Check sheet for the modelled part. Datum: model origin and axes. Units: mm. Coordinates: 2 decimals unless noted, no trailing zeros. Loops run counter-clockwise (first coordinate to the right, second up) from the corner with the lowest first, then second, coordinate; pieces in that order, holes last.
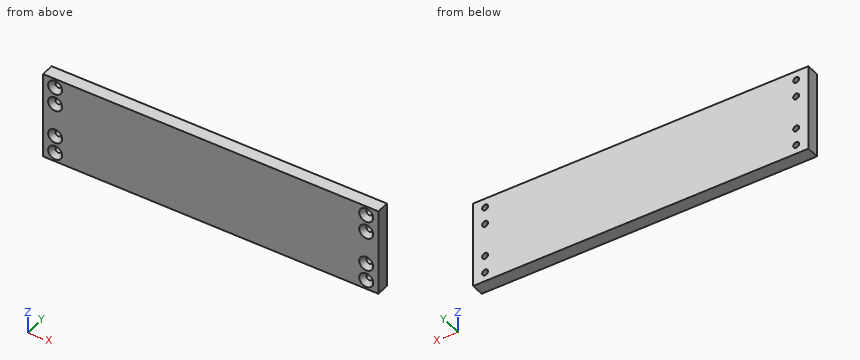
```python
from build123d import *

# Parameters (mm, degrees)
SKETCH1_W                                         = 166
SKETCH1_H                                         = 42.51
BOSS_EXTRUDE1_DEPTH                               = 6.35
F_4_CLEARANCE_HOLE1_D                             = 2.9464
CSK_FOR_4_FLAT_HEAD_SOCKET_CAP_SCREW1_D           = 2.9464
CSK_FOR_4_FLAT_HEAD_SOCKET_CAP_SCREW1_CSINK_D     = 6.9116702
CSK_FOR_4_FLAT_HEAD_SOCKET_CAP_SCREW1_CSINK_ANGLE = 82


with BuildPart() as part:
    # Sketch1 → Boss-Extrude1 (new body)
    with BuildSketch(Plane(origin=(0, 0, 0), x_dir=(1, 0, 0), z_dir=(0, 1, 0))):
        Rectangle(SKETCH1_W, SKETCH1_H)
    extrude(amount=BOSS_EXTRUDE1_DEPTH)

    # #4 Clearance Hole1 (through all)
    with Locations(Plane(origin=(0, 6.35, 0), x_dir=(1, 0, 0), z_dir=(0, 1, 0))):
        with Locations((-77, 8.255), (-77, 16.755), (77, 8.255), (77, 16.755)):
            Hole(F_4_CLEARANCE_HOLE1_D / 2)

    # CSK for #4 Flat Head Socket Cap Screw1 (through all)
    with Locations(Plane(origin=(0, 0, 0), x_dir=(-1, 0, 0), z_dir=(0, -1, 0))):
        with Locations((77, 8.255), (77, 16.755), (-77, 8.255), (-77, 16.755)):
            csk_for_4_flat_head_socket_cap_screw1 = CounterSinkHole(CSK_FOR_4_FLAT_HEAD_SOCKET_CAP_SCREW1_D / 2, CSK_FOR_4_FLAT_HEAD_SOCKET_CAP_SCREW1_CSINK_D / 2, counter_sink_angle=CSK_FOR_4_FLAT_HEAD_SOCKET_CAP_SCREW1_CSINK_ANGLE)

    # Mirror1: CSK for #4 Flat Head Socket Cap Screw1 across plane
    add(csk_for_4_flat_head_socket_cap_screw1.mirror(Plane.XY), mode=Mode.SUBTRACT)


solid = part.part
```
1) Section check A-A on x = -77. Enter the section's corners in (y, z) (3 decimals), plus the area to 3 significant figures.
Answer sheet:
outline: (0, -21.255) - (6.35, -21.255) - (6.35, -18.228) - (2.281, -18.228) - (0, -20.211) - close; (0, -13.299) - (2.281, -15.282) - (6.35, -15.282) - (6.35, -9.728) - (2.281, -9.728) - (0, -11.711) - close; (0, -4.799) - (2.281, -6.782) - (6.35, -6.782) - (6.35, 6.782) - (2.281, 6.782) - (0, 4.799) - close; (0, 11.711) - (2.281, 9.728) - (6.35, 9.728) - (6.35, 15.282) - (2.281, 15.282) - (0, 13.299) - close; (0, 20.211) - (2.281, 18.228) - (6.35, 18.228) - (6.35, 21.255) - (0, 21.255) - close
area: 177 mm2
2) Depth check by flat-ended pin: pin 1 (2.5 mm diameter, centred on x = 77, z = 16.755, fed in from -Y); pin 2 (4.5 mm diameter, centred on x = -77, z = 8.255, fed in from -Y). Enter the tip coordinate at first touch or a pass-through.
Answer sheet:
pin 1: passes through
pin 2: stops at y = 1.39
3) Scan lines: line 1 (Z direction, x = 77, y = 4.25) (3 decimals); line 2 (X direction, y = 4, z = 8.5); line 3 (X direction, y = 0.75, z = -8). Record each from-to range of solid material in increasing order.
Answer sheet:
line 1: z = -21.255 to -18.228, -15.282 to -9.728, -6.782 to 6.782, 9.728 to 15.282, 18.228 to 21.255
line 2: x = -83 to -78.45, -75.55 to 75.55, 78.45 to 83
line 3: x = -83 to -79.79, -74.21 to 74.21, 79.79 to 83
